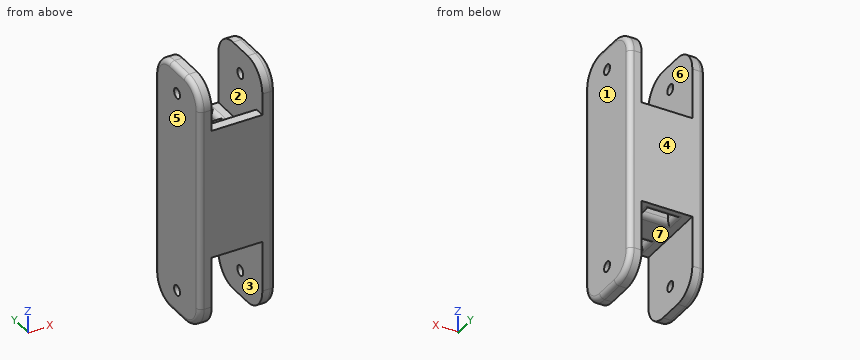
from build123d import *

# Parameters (mm, degrees)
BOTTOM_SECTION_BASE_SKETCH_W     = 15
BOTTOM_SECTION_BASE_SKETCH_H     = 15
BOTTOM_SECTION_EXTRUDE_DEPTH     = 50
HINGE_CUTOUT_SKETCH_W            = 10
HINGE_CUTOUT_SKETCH_H            = 15
HINGE_CUTOUT_EXTRUDED_CUT_DEPTH  = 15
HINGE_HOLE_SKETCH_R              = 1
HINGE_HOLE_EXTRUDED_CUT_DEPTH    = 53.737557774
HINGER_CORNER_FILLETS_R          = 5
STYLE_FILLETS_R                  = 1
ROUTING_HOLES_SKETCH_W           = 5
ROUTING_HOLES_SKETCH_H           = 2
ROUTING_HOLES_EXTRUDED_CUT_DEPTH = 52.112620751
BACKING_SKETCH_W                 = 10
BACKING_SKETCH_H                 = 2
BACKING_EXTRUDE_DEPTH            = 5.75
ROUTING_FILLETS_R                = 1


with BuildPart() as part:
    # Bottom Section Base Sketch → Bottom Section Extrude (new body)
    with BuildSketch(Plane.XY):
        Rectangle(BOTTOM_SECTION_BASE_SKETCH_W, BOTTOM_SECTION_BASE_SKETCH_H)
    extrude(amount=BOTTOM_SECTION_EXTRUDE_DEPTH)

    # Hinge Cutout Sketch → Hinge Cutout Extruded Cut (cut)
    with BuildSketch(Plane.XY):
        Rectangle(HINGE_CUTOUT_SKETCH_W, HINGE_CUTOUT_SKETCH_H)
    hinge_cutout_extruded_cut = extrude(amount=HINGE_CUTOUT_EXTRUDED_CUT_DEPTH, mode=Mode.SUBTRACT)

    # Hinge Hole Sketch → Hinge Hole Extruded Cut (cut, through all)
    with BuildSketch(Plane(origin=(7.5, 0, 0), x_dir=(0, 0, -1), z_dir=(1, 0, 0))):
        with Locations((-5, 0)):
            Circle(HINGE_HOLE_SKETCH_R)
    hinge_hole_extruded_cut = extrude(amount=-HINGE_HOLE_EXTRUDED_CUT_DEPTH, mode=Mode.SUBTRACT)

    # Hinge and Hole Cutout Mirror: Hinge Cutout Extruded Cut, Hinge Hole Extruded Cut across plane
    add(hinge_cutout_extruded_cut.mirror(Plane.XY.offset(25)), mode=Mode.SUBTRACT)
    add(hinge_hole_extruded_cut.mirror(Plane.XY.offset(25)), mode=Mode.SUBTRACT)

    # Hinger Corner Fillets
    hinger_corner_fillets_edges = [part.edges().sort_by_distance(p)[0] for p in [
        (6.25, -7.5, 0),
        (-6.25, 7.5, 0),
        (-6.25, -7.5, 50),
        (-6.25, 7.5, 50),
        (6.25, -7.5, 50),
        (-6.25, -7.5, 0),
        (6.25, 7.5, 0),
        (6.25, 7.5, 50),
    ]]
    fillet(hinger_corner_fillets_edges, radius=HINGER_CORNER_FILLETS_R)

    # Style Fillets
    style_fillets_edges = [part.edges().sort_by_distance(p)[0] for p in [
        (7.5, 0, 50),
        (7.5, 7.5, 25),
        (-7.5, 7.5, 25),
        (7.5, 0, 0),
        (7.5, -7.5, 25),
        (7.5, 6.035533906, 1.464466094),
        (7.5, -6.035533906, 1.464466094),
        (7.5, -6.035533906, 48.535533906),
        (7.5, 6.035533906, 48.535533906),
        (-7.5, -7.5, 25),
        (-7.5, 0, 50),
        (-7.5, 0, 0),
        (-7.5, -6.035533906, 1.464466094),
        (-7.5, 6.035533906, 1.464466094),
        (-7.5, 6.035533906, 48.535533906),
        (-7.5, -6.035533906, 48.535533906),
    ]]
    fillet(style_fillets_edges, radius=STYLE_FILLETS_R)

    # Routing Holes Sketch → Routing Holes Extruded Cut (cut, through all)
    with BuildSketch(Plane.XY):
        with Locations((0, 4.5)):
            Rectangle(ROUTING_HOLES_SKETCH_W, ROUTING_HOLES_SKETCH_H)
        with Locations((0, -4.5)):
            Rectangle(ROUTING_HOLES_SKETCH_W, ROUTING_HOLES_SKETCH_H)
    extrude(amount=ROUTING_HOLES_EXTRUDED_CUT_DEPTH, mode=Mode.SUBTRACT)

    # Backing Sketch → Backing Extrude (add)
    with BuildSketch(Plane.XY.offset(35)):
        with Locations((0, -6.5)):
            Rectangle(BACKING_SKETCH_W, BACKING_SKETCH_H)
    extrude(amount=BACKING_EXTRUDE_DEPTH)

    # Routing Fillets
    routing_fillets_edges = [part.edges().sort_by_distance(p)[0] for p in [
        (-2.5, -4.5, 35),
        (0, -3.5, 35),
        (2.5, -4.5, 35),
        (0, 5.5, 35),
        (2.5, 4.5, 35),
        (0, 3.5, 35),
        (-2.5, 4.5, 35),
        (-2.5, 4.5, 15),
        (0, 3.5, 15),
        (2.5, 4.5, 15),
        (0, 5.5, 15),
        (0, -5.5, 15),
        (2.5, -4.5, 15),
        (0, -3.5, 15),
        (-2.5, -4.5, 15),
    ]]
    fillet(routing_fillets_edges, radius=ROUTING_FILLETS_R)


solid = part.part
Can you work these out from the model? Positions are in its coordinate system, mm. Face numbers are marked on the shaded views. A direction names the side the tool comes from. Give positions to 0.01 mm unless a question says otherwise; leave off trailing zeros. Write each loop counter-clockwise with the first axis right and the second up, starting at its lowest first coordinate (ties: lowest second). Pieces come first, ordered by that corner, then holes. Notation, with made-up numbers: (75, 31) -> (81, 31) arc R5 ccw to (81, 37) -> close; hole circle Ø11 at (28, 62.5). An arc over 180 degrees is marked (long way). Answer as a JSON object with one key per item and string values. Group by question number.
Item 1: I'm going to push flat-ended pins straight in: P1, Ø3, axis at x = 2, y = 0.5, coming from the -Z side; P2, Ø1.5, axis at x = -5.5, y = -5, coming from the +Z side; P3, Ø1.6, axis at x = -0.5, y = -6, coming from the +Z side; P4, Ø1.8, axis at y = 0, z = 45, coming from the -X side. Where does each tip first touch, or does it pass through?
Item 2: Suppose I cut it at B-B (x = 1.25). Please give me the cut outline in (y, z), plus the area to 3 significant figures.
Item 3: We'd pull the mould along X, two halves only. Please class the marked faces 1, 2, 3 and 4: +X half, -X half, draft (parallel to the pull), parting line (faces both ways), or undercut.
Item 4: Suppose I cut it at D-D (z = 8.5). Please give me the cut outline in (x, y), plus the area to 3 significant figures.
Item 5: Suppose I cut it at C-C (z = 20). Please give me the cut outline in (x, y).
Item 6: For the marked faces 5, 6 and 7, which set-ups out of +Z, -Z, +X, -X, +Y, -Y let a thin tool reach every point of the face, with its end or its side?
Item 7: Please list where these lines run through material, in increasing order: line 1 (Y direction, x = 1, z = 19); line 2 (X direction, y = -3, z = 12.5); line 3 (Y direction, x = 5.65, z = 5). Write a range as [from, to].
Item 8: Suppose I cut it at A-A (y = 0). State how many separate pieces and enclosed holes the cut face has, plus the area to 3 significant figures.
Findings:
{
 "1": {"P1": "stops at z = 15", "P2": "stops at z = 49.68", "P3": "stops at z = 40.75", "P4": "passes through"},
 "2": {"outline": "(-7.5, 15) -> (-6.5, 15) arc R1 ccw to (-5.5, 16) -> (-5.5, 40.75) -> (-7.5, 40.75) -> close; (-3.5, 16) arc R1 ccw to (-2.5, 15) -> (2.5, 15) arc R1 ccw to (3.5, 16) -> (3.5, 34) arc R1 ccw to (2.5, 35) -> (-2.5, 35) arc R1 ccw to (-3.5, 34) -> close; (5.5, 16) arc R1 ccw to (6.5, 15) -> (7.5, 15) -> (7.5, 35) -> (6.5, 35) arc R1 ccw to (5.5, 34) -> close", "area": "230 mm²"},
 "3": {"face 1": "+X half", "face 2": "undercut", "face 3": "undercut", "face 4": "draft"},
 "4": {"outline": "(-7.5, -6.5) arc R1 ccw to (-6.5, -7.5) -> (-5, -7.5) -> (-5, 7.5) -> (-6.5, 7.5) arc R1 ccw to (-7.5, 6.5) -> close; (5, -7.5) -> (6.5, -7.5) arc R1 ccw to (7.5, -6.5) -> (7.5, 6.5) arc R1 ccw to (6.5, 7.5) -> (5, 7.5) -> close", "area": "74.1 mm²"},
 "5": {"outline": "(-7.5, -6.5) arc R1 ccw to (-6.5, -7.5) -> (6.5, -7.5) arc R1 ccw to (7.5, -6.5) -> (7.5, 6.5) arc R1 ccw to (6.5, 7.5) -> (-6.5, 7.5) arc R1 ccw to (-7.5, 6.5) -> close; hole (-2.5, -5.5) -> (2.5, -5.5) -> (2.5, -3.5) -> (-2.5, -3.5) -> close; hole (-2.5, 3.5) -> (2.5, 3.5) -> (2.5, 5.5) -> (-2.5, 5.5) -> close"},
 "6": {"face 5": "+Z, -Z, -X, +Y, -Y", "face 6": "+Z, +Y", "face 7": "-Z, +Y, -Y"},
 "7": {"line 1": "y = [-7.5, -5.5], [-3.5, 3.5], [5.5, 7.5]", "line 2": "x = [-7.5, -5], [5, 7.5]", "line 3": "y = [-7.5, -1], [1, 7.5]"},
 "8": {"separate pieces": "5", "enclosed holes": "0", "area": "429 mm²"}
}
